from build123d import *

# Parameters (mm, degrees)
SKETCH_1_W          = 20
SKETCH_1_H          = 40
SKETCH_1_W_2        = 16
SKETCH_1_H_2        = 36
EXTRUDE_1_DEPTH     = 315
SKETCH_2_R          = 2
CUT_EXTRUDE_1_DEPTH = 319.158765399
SKETCH_3_R          = 1.75
CUT_EXTRUDE_2_DEPTH = 319.158765399
SKETCH_5_R          = 1.75
CUT_EXTRUDE_4_DEPTH = 319.158765399


with BuildPart() as part:
    # 草图1 → 凸台-拉伸1 (new body)
    with BuildSketch(Plane.XY):
        with Locations((10, 20)):
            Rectangle(SKETCH_1_W, SKETCH_1_H)
        with Locations((10, 20)):
            Rectangle(SKETCH_1_W_2, SKETCH_1_H_2, mode=Mode.SUBTRACT)
    extrude(amount=EXTRUDE_1_DEPTH)

    # 草图2 → 切除-拉伸1 (cut, through all)
    with BuildSketch(Plane(origin=(20, 0, 0), x_dir=(0, 0, -1), z_dir=(1, 0, 0))):
        with Locations((-300, 30)):
            Circle(SKETCH_2_R)
        with Locations((-25, 28)):
            Circle(SKETCH_2_R)
    extrude(amount=-CUT_EXTRUDE_1_DEPTH, mode=Mode.SUBTRACT)

    # 草图3 → 切除-拉伸2 (cut, through all)
    with BuildSketch(Plane(origin=(0, 0, 0), x_dir=(-1, 0, 0), z_dir=(0, -1, 0))):
        with Locations(Location((-10, -305, 0), (0, 0, 90))):
            Circle(SKETCH_3_R)
        with Locations(Location((-10, -285, 0), (0, 0, 90))):
            Circle(SKETCH_3_R)
        with Locations(Location((-10, -265, 0), (0, 0, 90))):
            Circle(SKETCH_3_R)
        with Locations(Location((-10, -245, 0), (0, 0, 90))):
            Circle(SKETCH_3_R)
        with Locations(Location((-10, -225, 0), (0, 0, 90))):
            Circle(SKETCH_3_R)
        with Locations(Location((-10, -205, 0), (0, 0, 90))):
            Circle(SKETCH_3_R)
        with Locations(Location((-10, -185, 0), (0, 0, 90))):
            Circle(SKETCH_3_R)
        with Locations(Location((-10, -165, 0), (0, 0, 90))):
            Circle(SKETCH_3_R)
        with Locations(Location((-10, -145, 0), (0, 0, 90))):
            Circle(SKETCH_3_R)
        with Locations(Location((-10, -125, 0), (0, 0, 90))):
            Circle(SKETCH_3_R)
        with Locations(Location((-10, -105, 0), (0, 0, 90))):
            Circle(SKETCH_3_R)
        with Locations(Location((-10, -85, 0), (0, 0, 90))):
            Circle(SKETCH_3_R)
        with Locations(Location((-10, -65, 0), (0, 0, 90))):
            Circle(SKETCH_3_R)
        with Locations(Location((-10, -45, 0), (0, 0, 90))):
            Circle(SKETCH_3_R)
    extrude(amount=-CUT_EXTRUDE_2_DEPTH, mode=Mode.SUBTRACT)

    # 草图5 → 切除-拉伸4 (cut, through all)
    with BuildSketch(Plane(origin=(20, 0, 0), x_dir=(0, 0, -1), z_dir=(1, 0, 0))):
        with Locations((-305, 17.65)):
            Circle(SKETCH_5_R)
        with Locations((-285, 17.65)):
            Circle(SKETCH_5_R)
        with Locations((-265, 17.65)):
            Circle(SKETCH_5_R)
        with Locations((-245, 17.65)):
            Circle(SKETCH_5_R)
        with Locations((-225, 17.65)):
            Circle(SKETCH_5_R)
        with Locations((-205, 17.65)):
            Circle(SKETCH_5_R)
        with Locations((-185, 17.65)):
            Circle(SKETCH_5_R)
        with Locations((-165, 17.65)):
            Circle(SKETCH_5_R)
        with Locations((-145, 17.65)):
            Circle(SKETCH_5_R)
        with Locations((-125, 17.65)):
            Circle(SKETCH_5_R)
        with Locations((-105, 17.65)):
            Circle(SKETCH_5_R)
        with Locations((-85, 17.65)):
            Circle(SKETCH_5_R)
        with Locations((-65, 17.65)):
            Circle(SKETCH_5_R)
        with Locations((-45, 17.65)):
            Circle(SKETCH_5_R)
    extrude(amount=-CUT_EXTRUDE_4_DEPTH, mode=Mode.SUBTRACT)


solid = part.part
Read the model definition and answer for the solid it produces. Units are mm, in the model's axes. A direction names the side the tool comes from. Coordinates: 2 decimals unless noted, no trailing zeros. Write each loop counter-clockwise with the first axis right and the second up, starting at its lowest first coordinate (ties: lowest second). Pieces come first, ordered by that corner, then holes. Notation, with made-up numbers: (9.5, 57.25) -> (43.5, 57.25) arc R35 cw to (43.5, 91.25) -> close; hole circle Ø10 at (70, 25.5). An arc over 180 degrees is marked (long way). Return JSON: item names as keys, results as strings.
(1) The part is cut by section B-B on z = 92. Give the vertices of the cut face in (x, y), then the cut area to 3 significant figures.
Answers below:
{"outline": "(0, 0) -> (20, 0) -> (20, 40) -> (0, 40) -> close; hole (2, 2) -> (18, 2) -> (18, 38) -> (2, 38) -> close", "area": "224 mm^2"}
(2) This flat-tipped pin is pushed along its axis until it touches: P1, Ø5, axis at x = 6.5, y = 22, coming from the +Z side. Where does it stop, or does it pass through?
Answers below:
{"P1": "through"}
(3) For a pull along Y with two mould halves and no side action, classify faces 1 (the flat face through (10, 40, 155)), 2 (the flat face through (18, 20, 155)), 3 (the flat face through (1.8, 21.6, 315)) as pulls with the +Y half, pulls with the -Y half, needs draft (parallel to the pull), parting line crosses it, or undercut.
Answers below:
{"face 1": "pulls with the +Y half", "face 2": "undercut", "face 3": "needs draft"}
(4) The part is cut by section A-A on y = 22.5. Give the vertices of the cut face in (x, z), then the cut area to 3 significant figures.
Answers below:
{"outline": "(0, 0) -> (2, 0) -> (2, 315) -> (0, 315) -> close; (18, 0) -> (20, 0) -> (20, 315) -> (18, 315) -> close", "area": "1,260 mm^2"}
(5) Which of the six approach directions +Z, -Z, +X, -X, +Y, -Y give full straight-line access (tool end or side, diameter ignored) to faces 4 (the flat face through (10, 2, 155)), 5 (the flat face through (20, 20, 155))?
Answers below:
{"face 4": "+Z, -Z", "face 5": "+Z, -Z, +X, +Y, -Y"}
(6) Consider line 1 along Y through (x, z) = (18.7, 105); line 2 along Y through (x, z) = (3.75, 80); line 3 along X through (y, z) = (11, 189). Determine where each line is inside the solid, lowest interval first. Write a range as from..to.
Answers below:
{"line 1": "0..15.9, 19.4..40", "line 2": "0..2, 38..40", "line 3": "0..2, 18..20"}
